Read the model definition and answer for the solid it produces. Units are mm, in the model's axes. A direction names the side the tool comes from. Coordinates: 2 decimals unless noted, no trailing zeros. Loops run counter-clockwise (first coordinate to the right, second up) from the corner with the lowest first, then second, coordinate; pieces in that order, holes last.
Q1. Section C-C (y = 12.5) is taken. Give the vertices of the cut face in (x, z).
Q2. Flat-ended cylindrical pins translate along their axes: P1, Ø1.5, axis at y = 78.5, z = 4, coming from the +X side; P2, Ø6, axis at y = -21.5, z = 1, coming from the -X side; P3, Ø3, axis at y = 49, z = 5.5, coming from the +X side. Find the tip coordinate at first contact, or state that the pin passes through.
Q3. Straight lines are drawn through the part: line 1 (Y direction, x = 0.5, z = -9); line 2 (Y direction, x = -4, z = -7.75); line 3 (Y direction, x = 9, z = -2.5). For each, find the intervals that lie inside material, in ascending order.
Q4. Section D-D (x = 9.5) is taken. Give the vertices of the cut face in (y, z).
Q5. Section B-B (x = -14) is taken. Give the vertices of the cut face in (y, z), then the cut area to 3 significant figures.
Q6. Which of the six approach directions +Z, -Z, +X, -X, +Y, -Y give full straight-line access (tool end or side, diameter ignored) to faces 3 (the face through (-6, 104, -0.3)), 4 (the face through (6.25, 133, 0)), 5 (the face through (4, 69, 0)), 6 (the face through (8, 97, 4)), 7 (the face through (-0.2, -21.3, 6))?
Q7. The mould has two halves that part along Y. Classify faces 1 (the face through (17, -19, 0)), 2 (the face through (12.3, 32.7, -0.1)): pulls with the +Y half, pulls with the -Y half, needs draft (parallel to the pull), parting line crosses it, or undercut.
Q8. Section A-A (z = -8) is taken. Give the vertices of the cut face in (x, y), then the cut area to 3 significant figures.
from build123d import *

# Parameters (mm, degrees)
BOSS_EXTRUDE2_DEPTH = 10
BOSS_EXTRUDE3_DEPTH = 6
CUT_EXTRUDE1_START  = 4
CUT_EXTRUDE1_DEPTH  = 140.802456026


with BuildPart() as part:
    # Sketch1 → Boss-Extrude2 (new, symmetric)
    with BuildSketch(Plane.XY):
        with BuildLine():
            ThreePointArc((6.25, 130.825317547), (3.235238064, 132.074072829), (0, 132.5))
            Line((0, 132.5), (0, 126.25))
            ThreePointArc((0, 126.25), (4.419417382, 124.419417382), (6.25, 120))
            ThreePointArc((6.25, 120), (4.419417382, 115.580582618), (0, 113.75))
            Line((0, 113.75), (0, 107.5))
            ThreePointArc((0, 107.5), (4.253905297, 108.246094703), (8, 110.395313644))
            ThreePointArc((8, 110.395313644), (11.319231423, 114.696699141), (12.5, 120))
            ThreePointArc((12.5, 120), (10.825317547, 126.25), (6.25, 130.825317547))
        make_face()
        with BuildLine():
            Line((0, 126.25), (0, 132.5))
            ThreePointArc((0, 132.5), (-3.235238064, 132.074072829), (-6.25, 130.825317547))
            ThreePointArc((-6.25, 130.825317547), (-12.454392393, 121.066822444), (-8, 110.395313644))
            ThreePointArc((-8, 110.395313644), (-4.253905297, 108.246094703), (0, 107.5))
            Line((0, 107.5), (0, 113.75))
            ThreePointArc((0, 113.75), (-6.25, 120), (0, 126.25))
        make_face()
        with BuildLine():
            ThreePointArc((6.25, 130.825317547), (3.235238064, 132.074072829), (0, 132.5))
            Line((0, 132.5), (0, 126.25))
            ThreePointArc((0, 126.25), (4.419417382, 124.419417382), (6.25, 120))
            ThreePointArc((6.25, 120), (4.419417382, 115.580582618), (0, 113.75))
            Line((0, 113.75), (0, 107.5))
            ThreePointArc((0, 107.5), (4.253905297, 108.246094703), (8, 110.395313644))
            ThreePointArc((8, 110.395313644), (11.319231423, 114.696699141), (12.5, 120))
            ThreePointArc((12.5, 120), (10.825317547, 126.25), (6.25, 130.825317547))
        make_face()
        with BuildLine():
            Line((0, 126.25), (0, 132.5))
            ThreePointArc((0, 132.5), (-3.235238064, 132.074072829), (-6.25, 130.825317547))
            ThreePointArc((-6.25, 130.825317547), (-12.454392393, 121.066822444), (-8, 110.395313644))
            ThreePointArc((-8, 110.395313644), (-4.253905297, 108.246094703), (0, 107.5))
            Line((0, 107.5), (0, 113.75))
            ThreePointArc((0, 113.75), (-6.25, 120), (0, 126.25))
        make_face()
        with BuildLine():
            ThreePointArc((19.704607906, 7.261434244), (12.010617821, 17.226289779), (0, 21))
            Line((0, 21), (0, 16))
            ThreePointArc((0, 16), (11.313708499, 11.313708499), (16, 0))
            ThreePointArc((16, 0), (11.313708499, -11.313708499), (0, -16))
            Line((0, -16), (0, -21))
            ThreePointArc((0, -21), (9.541871197, -18.707022587), (17, -12.328828006))
            ThreePointArc((17, -12.328828006), (19.974984355, -6.480740698), (21, 0))
            ThreePointArc((21, 0), (20.673615625, 3.688037011), (19.704607906, 7.261434244))
        make_face()
        with BuildLine():
            Line((0, 16), (0, 21))
            ThreePointArc((0, 21), (-12.010617821, 17.226289779), (-19.704607906, 7.261434244))
            ThreePointArc((-19.704607906, 7.261434244), (-20.802683821, -2.871993361), (-17, -12.328828006))
            ThreePointArc((-17, -12.328828006), (-9.541871197, -18.707022587), (0, -21))
            Line((0, -21), (0, -16))
            ThreePointArc((0, -16), (-16, 0), (0, 16))
        make_face()
        with BuildLine():
            ThreePointArc((19.704607906, 7.261434244), (12.010617821, 17.226289779), (0, 21))
            Line((0, 21), (0, 16))
            ThreePointArc((0, 16), (11.313708499, 11.313708499), (16, 0))
            ThreePointArc((16, 0), (11.313708499, -11.313708499), (0, -16))
            Line((0, -16), (0, -21))
            ThreePointArc((0, -21), (9.541871197, -18.707022587), (17, -12.328828006))
            ThreePointArc((17, -12.328828006), (19.974984355, -6.480740698), (21, 0))
            ThreePointArc((21, 0), (20.673615625, 3.688037011), (19.704607906, 7.261434244))
        make_face()
        with BuildLine():
            Line((0, 16), (0, 21))
            ThreePointArc((0, 21), (-12.010617821, 17.226289779), (-19.704607906, 7.261434244))
            ThreePointArc((-19.704607906, 7.261434244), (-20.802683821, -2.871993361), (-17, -12.328828006))
            ThreePointArc((-17, -12.328828006), (-9.541871197, -18.707022587), (0, -21))
            Line((0, -21), (0, -16))
            ThreePointArc((0, -16), (-16, 0), (0, 16))
        make_face()
    extrude(amount=BOSS_EXTRUDE2_DEPTH, both=True)

    # Sketch1_7 → Boss-Extrude3 (add, symmetric)
    with BuildSketch(Plane.XY):
        with BuildLine():
            ThreePointArc((8, 110.395313644), (4.253905297, 108.246094703), (0, 107.5))
            Line((0, 107.5), (0, 21))
            ThreePointArc((0, 21), (12.010617821, 17.226289779), (19.704607906, 7.261434244))
            ThreePointArc((19.704607906, 7.261434244), (10.727396888, 40.791551261), (8, 75.395313644))
            Line((8, 75.395313644), (8, 110.395313644))
        make_face()
        with BuildLine():
            ThreePointArc((0, 107.5), (-4.253905297, 108.246094703), (-8, 110.395313644))
            Line((-8, 110.395313644), (-8, 75.395313644))
            ThreePointArc((-8, 75.395313644), (-10.727396888, 40.791551261), (-19.704607906, 7.261434244))
            ThreePointArc((-19.704607906, 7.261434244), (-12.010617821, 17.226289779), (0, 21))
            Line((0, 21), (0, 107.5))
        make_face()
        with BuildLine():
            ThreePointArc((17, -12.328828006), (9.541871197, -18.707022587), (0, -21))
            Line((0, -21), (0, -24.828828006))
            Line((0, -24.828828006), (17, -24.828828006))
            Line((17, -24.828828006), (17, -12.328828006))
        make_face()
        with BuildLine():
            ThreePointArc((0, -21), (-9.541871197, -18.707022587), (-17, -12.328828006))
            Line((-17, -12.328828006), (-17, -24.828828006))
            Line((-17, -24.828828006), (0, -24.828828006))
            Line((0, -24.828828006), (0, -21))
        make_face()
        with BuildLine():
            Line((6.25, 135.825317547), (0, 135.825317547))
            Line((0, 135.825317547), (0, 132.5))
            ThreePointArc((0, 132.5), (3.235238064, 132.074072829), (6.25, 130.825317547))
            Line((6.25, 130.825317547), (6.25, 135.825317547))
        make_face()
        with BuildLine():
            Line((0, 132.5), (0, 135.825317547))
            Line((0, 135.825317547), (-6.25, 135.825317547))
            Line((-6.25, 135.825317547), (-6.25, 130.825317547))
            ThreePointArc((-6.25, 130.825317547), (-3.235238064, 132.074072829), (0, 132.5))
        make_face()
    extrude(amount=BOSS_EXTRUDE3_DEPTH, both=True)

    # Sketch2 → Cut-Extrude1 (cut)
    with BuildSketch(Plane(origin=(0, 0, 0), x_dir=(0, 0, -1), z_dir=(1, 0, 0)).offset(CUT_EXTRUDE1_START)):
        with BuildLine():
            Line((4.310429138, 99.95992073), (3.689169265, 37.95992073))
            ThreePointArc((3.689169265, 37.95992073), (-0.350709206, 34.000200799), (-4.310429138, 38.04007927))
            Line((-4.310429138, 38.04007927), (-3.689169265, 100.04007927))
            ThreePointArc((-3.689169265, 100.04007927), (0.350709206, 103.999799201), (4.310429138, 99.95992073))
        make_face()
    cut_extrude1 = extrude(amount=CUT_EXTRUDE1_DEPTH, mode=Mode.SUBTRACT)

    # Mirror1: Cut-Extrude1 across plane
    add(cut_extrude1.mirror(Plane(origin=(0, 0, 0), x_dir=(0, 0, 1), z_dir=(1, 0, 0))), mode=Mode.SUBTRACT)


solid = part.part
Numbers:
1. outline: (-17.86, -6) - (-16.87, -6) - (-16.87, -10) - (-9.99, -10) - (-9.99, 10) - (-16.87, 10) - (-16.87, 6) - (-17.86, 6) - close; (9.99, -10) - (16.87, -10) - (16.87, -6) - (17.86, -6) - (17.86, 6) - (16.87, 6) - (16.87, 10) - (9.99, 10) - close
2. P1: stops at x = 8
2. P2: stops at x = -17
2. P3: stops at x = 9.7
3. line 1: y = -20.99 to -15.99, 15.99 to 20.99, 107.51 to 113.77, 126.23 to 132.49
3. line 2: y = -20.62 to -15.49, 15.49 to 20.62, 108.16 to 115.2, 124.8 to 131.84
3. line 3: y = -24.83 to -13.23, 13.23 to 35.15, 111.33 to 128.67
4. outline: (-24.83, -6) - (-18.73, -6) - (-18.73, -10) - (-12.87, -10) - (-12.87, 10) - (-18.73, 10) - (-18.73, 6) - (-24.83, 6) - close; (12.87, -10) - (18.73, -10) - (18.73, -6) - (49.01, -6) - (49.01, -3.8) - (37.96, -3.69) arc R4 cw to (38.04, 4.31) - (49.01, 4.2) - (49.01, 6) - (18.73, 6) - (18.73, 10) - (12.87, 10) - close; (111.88, -10) - (128.12, -10) - (128.12, 10) - (111.88, 10) - close
5. outline: (-24.83, -6) - (-15.65, -6) - (-15.65, -10) - (-7.75, -10) - (-7.75, 10) - (-15.65, 10) - (-15.65, 6) - (-24.83, 6) - close; (7.75, -10) - (15.65, -10) - (15.65, -6) - (25.53, -6) - (25.53, 6) - (15.65, 6) - (15.65, 10) - (7.75, 10) - close
5. area: 545 mm2
6. face 3: -X
6. face 4: +Z, -Z, +X, +Y
6. face 5: +X
6. face 6: +Z, -Z, +X
6. face 7: +Z, -Y
7. face 1: needs draft
7. face 2: undercut
8. outline: circle Ø42 at (0, 0); circle Ø25 at (0, 120); hole circle Ø32 at (0, 0); hole circle Ø12.5 at (0, 120)
8. area: 949 mm2
